```python
from build123d import *

# Parameters (mm, degrees)
CUT_EXTRUDE1_DEPTH      = 32.44305901
CUT_EXTRUDE1_DEPTH_BACK = 32.44305901
SKETCH2_R               = 3


with BuildPart() as part:
    # Sketch1 → Revolve1 (revolve)
    with BuildSketch(Plane.XY, mode=Mode.PRIVATE) as revolve1_sk:
        Polygon((-9.2075, 6.93899031), (-9.2075, 5.967196114), (-9.2075, 0), (-6.905893187, 0), (-6.905893187, 6.416213171), (-6.905893187, 7.390660798), (-10.285280241, 8.689390938), (-5.259867997, 11.200858424), (-8.980968211, 12.630912137), (-2.983991931, 16.129225704), (-2.983991931, 18.916244006), (-4.436960556, 19.474633476), (0, 21.979471408), (0, 25.578013153), (-3.25, 25.578013153), (-3.25, 21.491279951), (-8.434096868, 19.368086458), (-5.067424881, 16.708608808), (-11.404533468, 13.131062925), (-7.295164247, 11.551793791), (-12.931187167, 8.370038214), align=None)
    revolve(revolve1_sk.sketch.rotate(Axis((0, -7.059352361, 0), (0, 1, 0)), 270), axis=Axis((0, -7.059352361, 0), (0, 1, 0)))

    # Sketch2 → Cut-Extrude1 (cut, two sides: drawn at the far end of the back side and taken through both)
    with BuildSketch(Plane(origin=(0, 25.578013153, 0), x_dir=(1, 0, 0), z_dir=(0, 1, 0)).offset(-CUT_EXTRUDE1_DEPTH_BACK)):
        with Locations(Location((0, 0, 0), (0, 0, 90))):
            Circle(SKETCH2_R)
    extrude(amount=CUT_EXTRUDE1_DEPTH + CUT_EXTRUDE1_DEPTH_BACK, mode=Mode.SUBTRACT)


solid = part.part
```
Part model, mm, in its own coordinate system. A direction names the side the tool comes from. Round coordinates to 2 decimals unless told otherwise and drop trailing zeros. Loops run counter-clockwise (first coordinate to the right, second up) from the corner with the lowest first, then second, coordinate; pieces in that order, holes last.
Item 1: Drill centre lines: line 1 (X direction, y = 22.65, z = 0); line 2 (Y direction, x = -7.75, z = 0); line 3 (X direction, y = 2, z = -0.25). Where is each one in solid material? Low to high.
Item 2: Mould opens along Z. For faces 1 (the face through (-6.847, 3.747, 0.899)), 2 (the face through (-2.82, 7.008, -8.955)), 3 (the face through (-7, 0, -1)) say: +Z half, -Z half, draft (parallel to the pull), parting line (faces both ways), or undercut.
Item 3: Cut at B-B, the plane x = 9.75. State how many separate pieces and enclosed holes the cut face has, then the cut area to 3 significant figures.
Item 4: Cut at A-A, the plane y = 24. Give the cut face in (x, z), then the cut area to 3 significant figures.
Item 5: Cut at C-C, the plane y = 5. Give the cut face in (x, z) (1 decimal).
Item 6: 3-axis set-ups, long thin cutter, end or side, ignore diameter. For faces 4 (the face through (-0.9, 17.5, -2.86)), 5 (the face through (5.36, 11.29, 1.19)), 6 (the face through (1.978, 23.506, 2.579)), 7 (the face through (5.6, 3.42, 7.31)): which of +Z, -Z, +X, -X, +Y, -Y reach the whole face in a straight line?
Item 7: Drop flat-ended pins along their axis: P1, Ø4, axis at x = 6, z = -2.5, coming from the +Y side; P2, Ø2, axis at x = 0.5, z = 4, coming from the +Y side; P3, Ø7, axis at x = 0, z = 0, coming from the -Y side; P4, Ø3.5, axis at x = 0, z = 0, coming from the +Y side. Give the stop position or say it passes through.
A:
1. line 1: x = -3.25 to -3, 3 to 3.25
1. line 2: y = 0 to 7.72, 9.96 to 11.3, 11.73 to 12.16, 13.35 to 15.19, 18.83 to 19.65
1. line 3: x = -9.2 to -6.9, 6.9 to 9.2
2. face 1: undercut
2. face 2: parting line
2. face 3: draft
3. separate pieces: 2
3. enclosed holes: 1
3. area: 43.3 mm2
4. outline: circle Ø6.5 at (0, 0); hole circle Ø6 at (0, 0)
4. area: 4.91 mm2
5. outline: circle Ø18.4 at (0, 0); hole circle Ø13.8 at (0, 0)
6. face 4: +Y, -Y
6. face 5: none
6. face 6: +Y
6. face 7: -Y
7. P1: stops at y = 20.98
7. P2: stops at y = 25.58
7. P3: stops at y = 15.83
7. P4: passes through
